CAD build for the part. Positions are in the model's coordinates, mm. A direction names the side the tool comes from. Coordinates: 2 decimals unless noted, no trailing zeros. Order: outer loops, then holes, each group sorted by start corner. A loop starts at its lowest first (then second) coordinate and runs counter-clockwise, first axis right, second up. Notation, with made-up numbers: (57, 14.25) -> (95, 14.25) arc R3 ccw to (95, 19.25) -> close; hole circle Ø1 at (52, -4). An arc over 180 degrees is marked (long way). Use one line per item in the form item = value. Start each with the question number.
from build123d import *

# Parameters (mm, degrees)
F1_DEPTH      = 10
F2_R          = 2
F3_DEPTH      = 15.001
F3_DEPTH_BACK = 107.001


with BuildPart() as f1:
    # F0 (on Front) → F1 (new body)
    with BuildSketch(Plane.XZ):
        Polygon((-61, 170), (-61, 0), (61, 0), (61, 170), (46, 170), (46, 160), (51, 160), (51, 10), (0, 10), (-51, 10), (-51, 160), (-46, 160), (-46, 170), align=None)
    extrude(amount=F1_DEPTH)

    # F2 (on face) → F3 (cut, two sides)
    with BuildSketch(Plane.YZ.offset(-46)) as f3_sk:
        with Locations((-5, 165)):
            Circle(F2_R)
    extrude(amount=-F3_DEPTH, mode=Mode.SUBTRACT)
    extrude(f3_sk.sketch, amount=F3_DEPTH_BACK, mode=Mode.SUBTRACT)


solid = f1.part
1) Two-plate mould, pull along Z, no slides. Class faces 1 (the face through (-1, -5, 0)), 2 (the face through (48, -5, 160)), 3 (the face through (-53, -5, 170)), 4 (the face through (46, -4.9, 167.3)): released by +Z, released by -Z, zero draft, split by the parting line, or undercut.
2) Cut at D-D on x = -20.5. Give the cut face in (y, z), then the cut area to 3 significant figures.
3) Cut at C-C on z = 129. Give the cut face in (x, y), then the cut area to 3 significant figures.
4) Probe L1, parallel to X at y = -7.75, z = 104; L2, parallel to Y at x = 53.5, z = 165; L3, parallel to Z at x = 58, y = -5. List the from-to ranges inside material, lowest first.
5) Cut at B-B on y = -5. Give the cut face in (x, z), then the cut area to 3 significant figures.
6) Drop flat-ended pins along their axis: P1, Ø1.5, axis at x = -23.5, y = -9, coming from the +Z side; P2, Ø3.5, axis at y = -5, z = 165, coming from the +X side. Give the stop position or say it passes through.
7) 3-axis set-ups, long thin cutter, end or side, ignore diameter. For faces 5 (the face through (-46, -4.9, 162.7)), 6 (the face through (-61, -5, 86)), 7 (the face through (-49, -5, 160)): which of +Z, -Z, +X, -X, +Y, -Y reach the whole face in a straight line?
8) Cut at A-A on z = 165. Give the cut face in (x, y), then the cut area to 3 significant figures.
Values follow:
q1.face_1 = released by -Z
q1.face_2 = undercut
q1.face_3 = released by +Z
q1.face_4 = zero draft
q2.outline = (-10, 0) -> (0, 0) -> (0, 10) -> (-10, 10) -> close
q2.area = 100 mm^2
q3.outline = (-61, -10) -> (-51, -10) -> (-51, 0) -> (-61, 0) -> close; (51, -10) -> (61, -10) -> (61, 0) -> (51, 0) -> close
q3.area = 200 mm^2
q4.L1 = -61 to -51, 51 to 61
q4.L2 = -10 to -7, -3 to 0
q4.L3 = 0 to 163, 167 to 170
q5.outline = (-61, 0) -> (61, 0) -> (61, 163) -> (46, 163) -> (46, 160) -> (51, 160) -> (51, 10) -> (-51, 10) -> (-51, 160) -> (-46, 160) -> (-46, 163) -> (-61, 163) -> close; (-61, 167) -> (-46, 167) -> (-46, 170) -> (-61, 170) -> close; (46, 167) -> (61, 167) -> (61, 170) -> (46, 170) -> close
q5.area = 4,400 mm^2
q6.P1 = 10
q6.P2 = through
q7.face_5 = +Z, +Y, -Y
q7.face_6 = +Z, -Z, -X, +Y, -Y
q7.face_7 = +Y, -Y
q8.outline = (-61, -10) -> (-46, -10) -> (-46, -7) -> (-61, -7) -> close; (-61, -3) -> (-46, -3) -> (-46, 0) -> (-61, 0) -> close; (46, -10) -> (61, -10) -> (61, -7) -> (46, -7) -> close; (46, -3) -> (61, -3) -> (61, 0) -> (46, 0) -> close
q8.area = 180 mm^2
